Design review of the part built by this model. Coordinates are the model's own, in mm. Round coordinates to 2 decimals unless told otherwise and drop trailing zeros. Order: outer loops, then holes, each group sorted by start corner. A loop starts at its lowest first (then second) coordinate and runs counter-clockwise, first axis right, second up.
from build123d import *

# Parameters (mm, degrees)
SKETCH1_R           = 1.5875
SKETCH1_R_2         = 3.556
SKETCH1_R_3         = 1.016
BOSS_EXTRUDE1_DEPTH = 3.175


with BuildPart() as part:
    # Sketch1 → Boss-Extrude1 (new body)
    with BuildSketch(Plane(origin=(0, 0, 0), x_dir=(1, 0, 0), z_dir=(0, 1, 0))):
        with BuildLine():
            Line((-64.92875, 9.417234118), (-2.8575, 18.834468236))
            ThreePointArc((-2.8575, 18.834468236), (19.05, 0), (-2.8575, -18.834468236))
            Line((-2.8575, -18.834468236), (-64.92875, -9.417234118))
            ThreePointArc((-64.92875, -9.417234118), (-73.025, 0), (-64.92875, 9.417234118))
        make_face()
        with Locations((-63.5, 0)):
            Circle(SKETCH1_R, mode=Mode.SUBTRACT)
        Circle(SKETCH1_R_2, mode=Mode.SUBTRACT)
        with Locations((0, 12.7)):
            Circle(SKETCH1_R_3, mode=Mode.SUBTRACT)
        with Locations((12.7, 0)):
            Circle(SKETCH1_R_3, mode=Mode.SUBTRACT)
        with Locations((0, -12.7)):
            Circle(SKETCH1_R_3, mode=Mode.SUBTRACT)
        with Locations((-12.7, 0)):
            Circle(SKETCH1_R_3, mode=Mode.SUBTRACT)
    extrude(amount=BOSS_EXTRUDE1_DEPTH)


solid = part.part
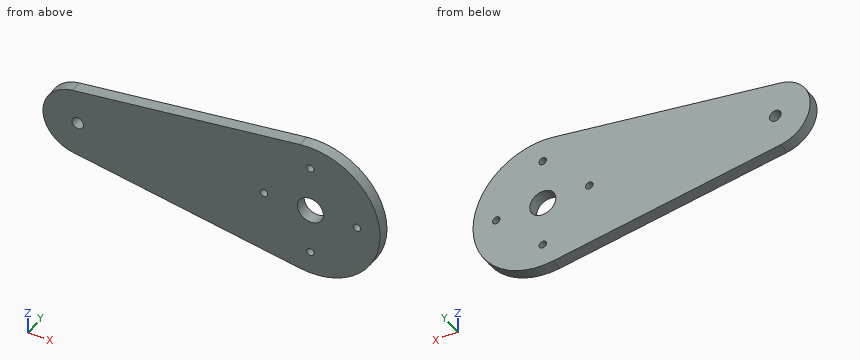
1) Take a section at C-C on x = 12.7. Give the boundary of the cut face in (y, z) (3 decimals), plus the area to 3 significant figures.
Results:
outline: (0, -14.199) - (3.175, -14.199) - (3.175, -1.016) - (0, -1.016) - close; (0, 1.016) - (3.175, 1.016) - (3.175, 14.199) - (0, 14.199) - close
area: 83.7 mm2
2) Clearance check with flat-ended pins moving along their axes: P1, Ø2.5, axis at x = -12.7, z = 0, coming from the +Y side (3 decimals); P2, Ø6.5, axis at x = 0, z = 0, coming from the +Y side; P3, Ø1.5, axis at x = -59, y = 1.5, coming from the -Z side. State where each tip first meets the part, or that it passes through.
Results:
P1: stops at y = 3.175
P2: passes through
P3: stops at z = -10.43
3) Take a section at D-D on z = 12.7. Give the boundary of the cut face in (x, y) (3 decimals), plus the area to 3 significant figures.
Results:
outline: (-43.291, 0) - (-1.016, 0) - (-1.016, 3.175) - (-43.291, 3.175) - close; (1.016, 0) - (14.199, 0) - (14.199, 3.175) - (1.016, 3.175) - close
area: 176 mm2
4) Take a section at A-A on z = 0. State how many separate pieces and enclosed holes the cut face has, plus the area to 3 significant figures.
Results:
separate pieces: 5
enclosed holes: 0
area: 247 mm2
5) To check wall thickness, follow line 1 along Z through (x, y) = (0, 1.2); line 2 along Z through (x, y) = (-12.7, 1.8); line 3 along X through (y, z) = (0.85, -3). State the ranges of each line that lie inside material, in increasing order.
Results:
line 1: z = -19.05 to -13.72, -11.68 to -3.56, 3.56 to 11.68, 13.72 to 19.05
line 2: z = -17.34 to -1.02, 1.02 to 17.34
line 3: x = -72.54 to -1.91, 1.91 to 18.81
